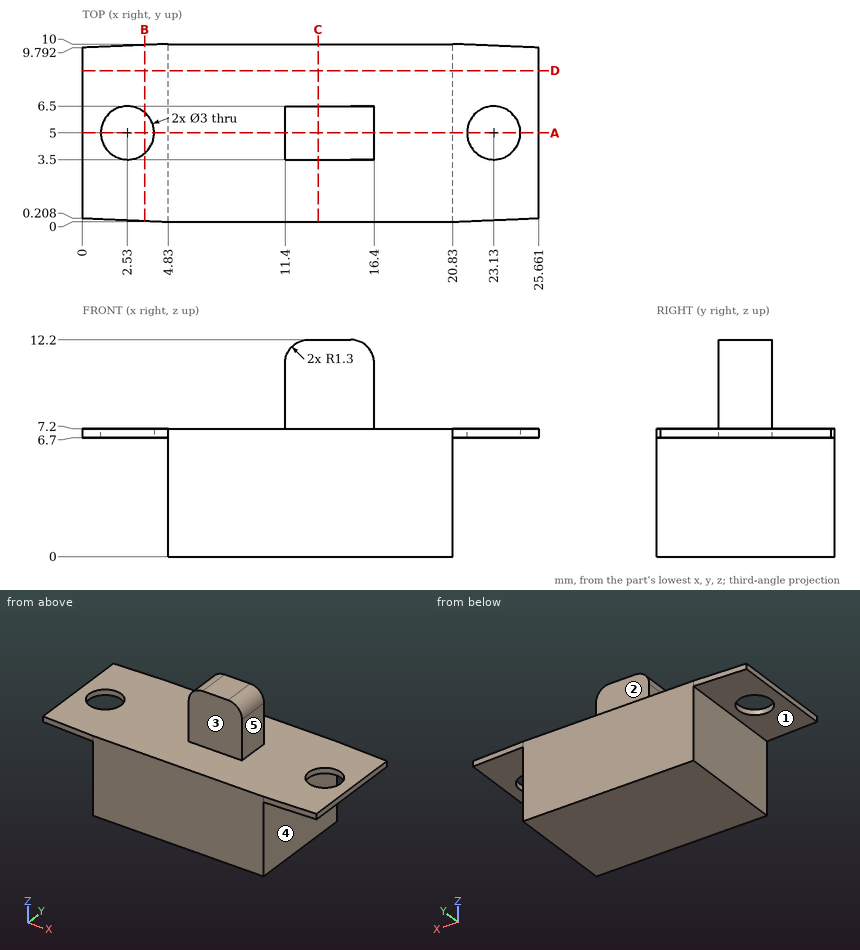
Geometry check sheet. Reference: drawing and pictorial views, mm from the part's lowest x, y, z. A direction names the side the tool comes from. Round coordinates to 2 decimals unless told otherwise and drop trailing zeros. Loops run counter-clockwise (first coordinate to the right, second up) from the corner with the lowest first, then second, coordinate; pieces in that order, holes last. Notation, with made-up numbers: (83, 18) - (98, 18) arc R25 ccw to (98, 50) - close; hole circle Ø9 at (9, -34.5). An arc over 180 degrees is marked (long way). One line per question, with ' | ' between items. Start each with the question number.
1. Cross-section at D-D on y = 8.5. Record the cut outline in (x, z).
2. Scan lines: line 1 (Z direction, x = 7, y = 8.75); line 2 (Z direction, x = 21.25, y = 5.5); line 3 (Y direction, x = 12.75, z = 10). Record each from-to range of solid material in increasing order. Write a range as [from, to].
3. Tool access check on the marked faces 1, 2, 3, 4 and 5. Record the directions out of +Z, -Z, +X, -X, +Y, -Y that give a thin tool (end or side, any length) a straight path to the whole face; none if there is none.
4. Cross-section at C-C on x = 13.25. Record the cut outline in (y, z), then the cut area to 3 significant figures.
5. Depth check by flat-ended pin: pin 1 (1.8 mm diameter, centred on x = 2.53, y = 5, fed in from +Z); pin 2 (1.4 mm diameter, centred on x = 3, y = 2.5, fed in from -Z); pin 3 (2.5 mm diameter, centred on x = 14.5, z = 8.5, fed in from +Y); pin 4 (2.5 mm diameter, centred on y = 4.5, z = 9, fed in from -X). Enter the tip coordinate at first touch or a pass-through.
6. Cross-section at A-A on y = 5. Record the cut outline in (x, z).
7. Cross-section at B-B on x = 3.5. Record the cut outline in (y, z) (1 decimal).
Taken from the geometry:
1) outline: (0, 6.7) - (4.83, 6.7) - (4.83, 0) - (20.83, 0) - (20.83, 6.7) - (25.66, 6.7) - (25.66, 7.2) - (0, 7.2) - close
2) line 1: [0, 7.2] | line 2: [6.7, 7.2] | line 3: [3.5, 6.5]
3) face 1: -Z, -X, +Y, -Y | face 2: +Z, +X, -X, +Y | face 3: +Z, +X, -X, -Y | face 4: -Z, +X, +Y, -Y | face 5: +Z, +X, +Y, -Y
4) outline: (0, 0) - (10, 0) - (10, 7.2) - (6.5, 7.2) - (6.5, 12.2) - (3.5, 12.2) - (3.5, 7.2) - (0, 7.2) - close | area: 87.0 mm²
5) pin 1: through | pin 2: z = 6.7 | pin 3: y = 6.5 | pin 4: x = 11.4
6) outline: (0, 6.7) - (1.03, 6.7) - (1.03, 7.2) - (0, 7.2) - close; (4.03, 6.7) - (4.83, 6.7) - (4.83, 0) - (20.83, 0) - (20.83, 6.7) - (21.63, 6.7) - (21.63, 7.2) - (16.4, 7.2) - (16.4, 10.9) arc R1.3 ccw to (15.1, 12.2) - (12.7, 12.2) arc R1.3 ccw to (11.4, 10.9) - (11.4, 7.2) - (4.03, 7.2) - close; (24.63, 6.7) - (25.66, 6.7) - (25.66, 7.2) - (24.63, 7.2) - close
7) outline: (0.1, 6.7) - (3.9, 6.7) - (3.9, 7.2) - (0.1, 7.2) - close; (6.1, 6.7) - (9.9, 6.7) - (9.9, 7.2) - (6.1, 7.2) - close
